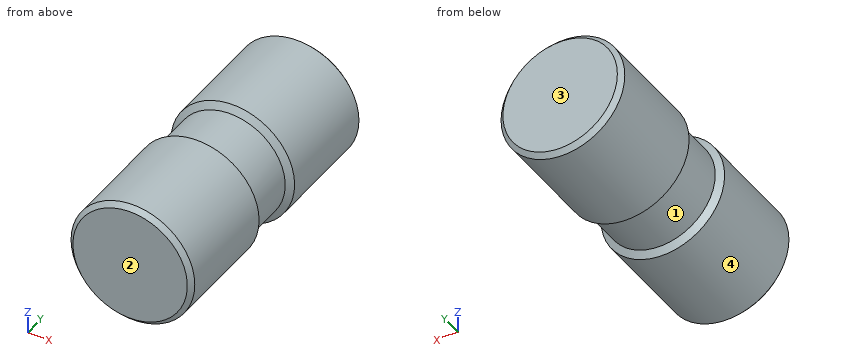
from build123d import *

# Parameters (mm, degrees)
F2_SIZE = 1.4


with BuildPart() as f1:
    # F0 (on Top) → F1 (revolve)
    with BuildSketch(Plane.XY):
        Polygon((0, -42.5), (0, 42.5), (-18.7, 42.5), (-18.7, 8.900415), (-16.7, 7.5), (-16.7, -7.5), (-18.7, -8.900415), (-18.7, -42.5), align=None)
    revolve(axis=Axis((0, 0, 0), (0, -1, 0)))

    # F2
    f2_edges = [f1.edges().sort_by_distance(p)[0] for p in [
        (18.7, 42.5, 0),
        (18.7, -42.5, 0),
    ]]
    chamfer(f2_edges, length=F2_SIZE)


solid = f1.part
Here's how the part is built. I have some questions about the finished solid (model axes, mm). Face numbers are marked on the shaded views. Round coordinates to 2 decimals unless told otherwise and drop trailing zeros. Order: outer loops, then holes, each group sorted by start corner. A loop starts at its lowest first (then second) coordinate and runs counter-clockwise, first axis right, second up. Notation, with made-up numbers: M 56.5,-34.5 L 89.5,-34.5 A11 ccw 89.5,-19.5 Z; hole C -28.5,70.5 d7. An arc over 180 degrees is marked long. Return JSON: item names as keys, results as strings. Group by question number.
1. If we mould it in two halves opening along Y, with no side actions, what happens to the marked faces 1, 2, 3 and 4? For each: pulls with the +Y half, pulls with the -Y half, needs draft (parallel to the pull), parting line crosses it, or undercut.
2. If we section it at C-C on y = -10: List the corners of the cut face in (x, z) for me, then the cut area to 3 significant figures.
3. Please list where these lines run through material, in increasing order: probe 1 along Y at (x, z) = (-4, 17); probe 2 along Y at (x, z) = (-14.5, 11); probe 3 along Z at (x, y) = (3.5, 36).
4. If we section it at A-A on z = 0: List the corners of the cut face in (x, y) for me, then the cut area to 3 significant figures.
5. If we section it at B-B on x = 0: List the corners of the cut face in (y, z) for me, then the cut area to 3 significant figures.
6. I'm going to push flat-ended pins straight in: pin 1 Ø1 at (y, z) = (5, 8.5) entering from -X; pin 2 Ø4 at (y, z) = (13.5, -14.5) entering from +X; pin 3 Ø2 at (x, y) = (-2.5, 28.5) entering from -Z. Where does each tip first touch, or does it pass through?
Reply:
{
 "1": {"face 1": "undercut", "face 2": "pulls with the -Y half", "face 3": "pulls with the +Y half", "face 4": "needs draft"},
 "2": {"outline": "C 0,0 d37.4", "area": "1,100 mm^2"},
 "3": {"probe 1": "-42.34 to -8.04, 8.04 to 42.34", "probe 2": "-41.6 to -8.55, 8.55 to 41.6", "probe 3": "-18.37 to 18.37"},
 "4": {"outline": "M -18.7,-41.1 L -17.3,-42.5 L 17.3,-42.5 L 18.7,-41.1 L 18.7,-8.9 L 16.7,-7.5 L 16.7,7.5 L 18.7,8.9 L 18.7,41.1 L 17.3,42.5 L -17.3,42.5 L -18.7,41.1 L -18.7,8.9 L -16.7,7.5 L -16.7,-7.5 L -18.7,-8.9 Z", "area": "3,110 mm^2"},
 "5": {"outline": "M -42.5,-17.3 L -41.1,-18.7 L -8.9,-18.7 L -7.5,-16.7 L 7.5,-16.7 L 8.9,-18.7 L 41.1,-18.7 L 42.5,-17.3 L 42.5,17.3 L 41.1,18.7 L 8.9,18.7 L 7.5,16.7 L -7.5,16.7 L -8.9,18.7 L -41.1,18.7 L -42.5,17.3 Z", "area": "3,110 mm^2"},
 "6": {"pin 1": "x = -14.66", "pin 2": "x = 13.91", "pin 3": "z = -18.64"}
}
